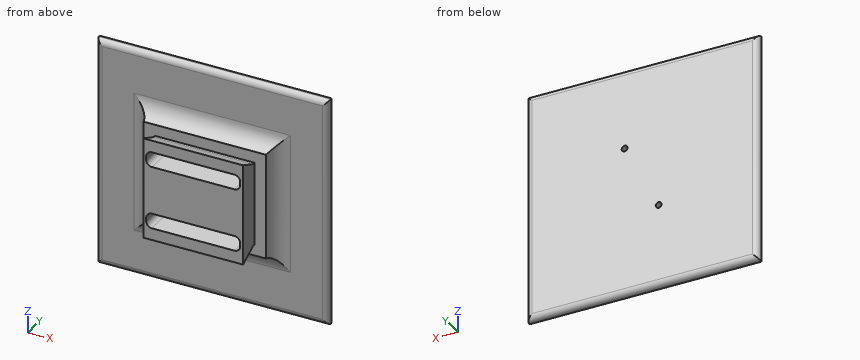
```python
from build123d import *

# Parameters (mm, degrees)
SKETCH1_W                  = 53.594
SKETCH1_H                  = 46.99
BOSS_EXTRUDE1_DEPTH        = 12.7
CUT_EXTRUDE1_DEPTH         = 62.251008522
SKETCH3_W                  = 4.953
SKETCH3_H                  = 9.653808373
CUT_EXTRUDE2_DEPTH         = 56.564640816
SKETCH4_W                  = 53.594
SKETCH4_H                  = 46.99
BOSS_EXTRUDE2_DEPTH        = 3.175
SKETCH5_W                  = 101.6
SKETCH5_H                  = 101.6
BOSS_EXTRUDE3_DEPTH        = 4.7625
FILLET1_R                  = 7.62
SKETCH6_W                  = 41.148
SKETCH6_H                  = 34.415052436
CUT_EXTRUDE3_DEPTH         = 15.875
F_2_6_2_6_DIAMETER_HOLE1_D = 2.6
FILLET2_R                  = 2.54
FILLET3_R                  = 2.54
FILLET4_R                  = 2.54
BOSS_EXTRUDE4_REACH        = 76.747
SKETCH9_W                  = 41.148
SKETCH9_H                  = 21.115558174
FILLET5_R                  = 2.54


with BuildPart() as part:
    # Sketch1 → Boss-Extrude1 (new body)
    with BuildSketch(Plane(origin=(0, 0, 0), x_dir=(1, 0, 0), z_dir=(0, 1, 0))):
        Rectangle(SKETCH1_W, SKETCH1_H)
    extrude(amount=BOSS_EXTRUDE1_DEPTH)

    # Sketch2 → Cut-Extrude1 (cut, through all)
    with BuildSketch(Plane(origin=(-26.797, 0, -3.302), x_dir=(0, 0, -1), z_dir=(1, 0, 0))):
        Polygon((-25.781, 0), (-21.779526218, 8.503564639), (-21.779526218, 9.653808373), (-26.797, 9.653808373), (-26.797, 0), align=None)
        Polygon((19.177, 0), (20.193, 0), (20.193, 9.653808373), (15.175526218, 9.653808373), (15.175526218, 8.503564639), align=None)
    extrude(amount=CUT_EXTRUDE1_DEPTH, mode=Mode.SUBTRACT)

    # Sketch3 → Cut-Extrude2 (cut, through all)
    with BuildSketch(Plane.XY.offset(23.495)):
        with Locations((-24.3205, 4.826904187)):
            Rectangle(SKETCH3_W, SKETCH3_H)
        with Locations((24.3205, 4.826904187)):
            Rectangle(SKETCH3_W, SKETCH3_H)
    extrude(amount=-CUT_EXTRUDE2_DEPTH, mode=Mode.SUBTRACT)

    # Sketch4 → Boss-Extrude2 (add)
    with BuildSketch(Plane(origin=(0, 12.7, 0), x_dir=(1, 0, 0), z_dir=(0, 1, 0))):
        Rectangle(SKETCH4_W, SKETCH4_H)
    extrude(amount=BOSS_EXTRUDE2_DEPTH)

    # Sketch5 → Boss-Extrude3 (add)
    with BuildSketch(Plane(origin=(0, 15.875, 0), x_dir=(1, 0, 0), z_dir=(0, 1, 0))):
        Rectangle(SKETCH5_W, SKETCH5_H)
    extrude(amount=BOSS_EXTRUDE3_DEPTH)

    # Fillet1
    # the kernel refuses this fillet: 7.62 mm, written as the material it adds along each edge
    with BuildSketch(Plane(origin=(-26.797, 15.875, -23.495), x_dir=(-1, 0, 0), z_dir=(0, 0, 1)), Plane(origin=(26.797, 15.875, 23.495), x_dir=(1, 0, 0), z_dir=(0, 0, -1))) as fillet1_piece_1:
        with BuildLine():
            CenterArc((7.490509671, 7.62), FILLET1_R, 190.577809731, 79.422190269)
            Line((0, 6.221191627), (-0.149810193, 6.19321546))
            ThreePointArc((-0.149810193, 6.19321546), (-0.1524, 3.110595814), (-0.1524, 0))
            Line((-0.1524, 0), (0, -0.1524))
            Line((0, -0.1524), (7.490509671, -0.1524))
            Line((7.490509671, -0.1524), (7.490509671, 0))
        make_face()
    extrude(amount=46.99)
    with BuildSketch(Plane(origin=(26.797, 15.875, -23.495), x_dir=(0, 0, -1), z_dir=(-1, 0, 0)), Plane(origin=(-26.797, 15.875, 23.495), x_dir=(0, 0, 1), z_dir=(1, 0, 0))) as fillet1_piece_2:
        with BuildLine():
            CenterArc((7.490509671, 7.62), FILLET1_R, 190.577809731, 79.422190269)
            Line((0, 6.221191627), (-0.149810193, 6.19321546))
            ThreePointArc((-0.149810193, 6.19321546), (-0.1524, 3.110595814), (-0.1524, 0))
            Line((-0.1524, 0), (0, -0.1524))
            Line((0, -0.1524), (7.490509671, -0.1524))
            Line((7.490509671, -0.1524), (7.490509671, 0))
        make_face()
    extrude(amount=53.594)
    with BuildSketch(Plane(origin=(26.797, 15.875, -23.495), x_dir=(0, 0, -1), z_dir=(-1, 0, 0))) as fillet1_piece_3a_section:
        with BuildLine():
            CenterArc((7.490509671, 7.62), FILLET1_R, 190.577809731, 79.422190269)
            Line((0, 6.221191627), (-0.149810193, 6.19321546))
            ThreePointArc((-0.149810193, 6.19321546), (-0.1524, 3.110595814), (-0.1524, 0))
            Line((-0.1524, 0), (0, -0.1524))
            Line((0, -0.1524), (7.490509671, -0.1524))
            Line((7.490509671, -0.1524), (7.490509671, 0))
        make_face()
    fillet1_piece_3a = extrude(amount=72.320274178, mode=Mode.PRIVATE)
    fillet1_piece_3a = split(fillet1_piece_3a, bisect_by=Plane(origin=(-26.797, 15.875, -23.495), z_dir=(-1, 0, 0)), keep=Keep.TOP, mode=Mode.PRIVATE)
    with BuildSketch(Plane(origin=(-26.797, 15.875, -42.221274178), x_dir=(-1, 0, 0), z_dir=(0, 0, 1))) as fillet1_piece_3b_section:
        with BuildLine():
            CenterArc((7.490509671, 7.62), FILLET1_R, 190.577809731, 79.422190269)
            Line((0, 6.221191627), (-0.149810193, 6.19321546))
            ThreePointArc((-0.149810193, 6.19321546), (-0.1524, 3.110595814), (-0.1524, 0))
            Line((-0.1524, 0), (0, -0.1524))
            Line((0, -0.1524), (7.490509671, -0.1524))
            Line((7.490509671, -0.1524), (7.490509671, 0))
        make_face()
    fillet1_piece_3b = extrude(amount=65.716274178, mode=Mode.PRIVATE)
    fillet1_piece_3b = split(fillet1_piece_3b, bisect_by=Plane(origin=(-26.797, 15.875, -23.495), z_dir=(0, 0, -1)), keep=Keep.TOP, mode=Mode.PRIVATE)
    fillet1_piece_3 = fillet1_piece_3a & fillet1_piece_3b
    add(fillet1_piece_3)
    with BuildSketch(Plane(origin=(-45.523274178, 15.875, 23.495), x_dir=(0, 0, 1), z_dir=(1, 0, 0))) as fillet1_piece_4a_section:
        with BuildLine():
            CenterArc((7.490509671, 7.62), FILLET1_R, 190.577809731, 79.422190269)
            Line((0, 6.221191627), (-0.149810193, 6.19321546))
            ThreePointArc((-0.149810193, 6.19321546), (-0.1524, 3.110595814), (-0.1524, 0))
            Line((-0.1524, 0), (0, -0.1524))
            Line((0, -0.1524), (7.490509671, -0.1524))
            Line((7.490509671, -0.1524), (7.490509671, 0))
        make_face()
    fillet1_piece_4a = extrude(amount=72.320274178, mode=Mode.PRIVATE)
    fillet1_piece_4a = split(fillet1_piece_4a, bisect_by=Plane(origin=(-26.797, 15.875, 23.495), z_dir=(-1, 0, 0)), keep=Keep.TOP, mode=Mode.PRIVATE)
    with BuildSketch(Plane(origin=(-26.797, 15.875, -23.495), x_dir=(-1, 0, 0), z_dir=(0, 0, 1))) as fillet1_piece_4b_section:
        with BuildLine():
            CenterArc((7.490509671, 7.62), FILLET1_R, 190.577809731, 79.422190269)
            Line((0, 6.221191627), (-0.149810193, 6.19321546))
            ThreePointArc((-0.149810193, 6.19321546), (-0.1524, 3.110595814), (-0.1524, 0))
            Line((-0.1524, 0), (0, -0.1524))
            Line((0, -0.1524), (7.490509671, -0.1524))
            Line((7.490509671, -0.1524), (7.490509671, 0))
        make_face()
    fillet1_piece_4b = extrude(amount=65.716274178, mode=Mode.PRIVATE)
    fillet1_piece_4b = split(fillet1_piece_4b, bisect_by=Plane(origin=(-26.797, 15.875, 23.495), z_dir=(0, 0, 1)), keep=Keep.TOP, mode=Mode.PRIVATE)
    fillet1_piece_4 = fillet1_piece_4a & fillet1_piece_4b
    add(fillet1_piece_4)
    with BuildSketch(Plane(origin=(26.797, 15.875, 23.495), x_dir=(1, 0, 0), z_dir=(0, 0, -1))) as fillet1_piece_5a_section:
        with BuildLine():
            CenterArc((7.490509671, 7.62), FILLET1_R, 190.577809731, 79.422190269)
            Line((0, 6.221191627), (-0.149810193, 6.19321546))
            ThreePointArc((-0.149810193, 6.19321546), (-0.1524, 3.110595814), (-0.1524, 0))
            Line((-0.1524, 0), (0, -0.1524))
            Line((0, -0.1524), (7.490509671, -0.1524))
            Line((7.490509671, -0.1524), (7.490509671, 0))
        make_face()
    fillet1_piece_5a = extrude(amount=65.716274178, mode=Mode.PRIVATE)
    fillet1_piece_5a = split(fillet1_piece_5a, bisect_by=Plane(origin=(26.797, 15.875, -23.495), z_dir=(0, 0, -1)), keep=Keep.TOP, mode=Mode.PRIVATE)
    with BuildSketch(Plane(origin=(45.523274178, 15.875, -23.495), x_dir=(0, 0, -1), z_dir=(-1, 0, 0))) as fillet1_piece_5b_section:
        with BuildLine():
            CenterArc((7.490509671, 7.62), FILLET1_R, 190.577809731, 79.422190269)
            Line((0, 6.221191627), (-0.149810193, 6.19321546))
            ThreePointArc((-0.149810193, 6.19321546), (-0.1524, 3.110595814), (-0.1524, 0))
            Line((-0.1524, 0), (0, -0.1524))
            Line((0, -0.1524), (7.490509671, -0.1524))
            Line((7.490509671, -0.1524), (7.490509671, 0))
        make_face()
    fillet1_piece_5b = extrude(amount=72.320274178, mode=Mode.PRIVATE)
    fillet1_piece_5b = split(fillet1_piece_5b, bisect_by=Plane(origin=(26.797, 15.875, -23.495), z_dir=(1, 0, 0)), keep=Keep.TOP, mode=Mode.PRIVATE)
    fillet1_piece_5 = fillet1_piece_5a & fillet1_piece_5b
    add(fillet1_piece_5)
    with BuildSketch(Plane(origin=(-26.797, 15.875, 23.495), x_dir=(0, 0, 1), z_dir=(1, 0, 0))) as fillet1_piece_6a_section:
        with BuildLine():
            CenterArc((7.490509671, 7.62), FILLET1_R, 190.577809731, 79.422190269)
            Line((0, 6.221191627), (-0.149810193, 6.19321546))
            ThreePointArc((-0.149810193, 6.19321546), (-0.1524, 3.110595814), (-0.1524, 0))
            Line((-0.1524, 0), (0, -0.1524))
            Line((0, -0.1524), (7.490509671, -0.1524))
            Line((7.490509671, -0.1524), (7.490509671, 0))
        make_face()
    fillet1_piece_6a = extrude(amount=72.320274178, mode=Mode.PRIVATE)
    fillet1_piece_6a = split(fillet1_piece_6a, bisect_by=Plane(origin=(26.797, 15.875, 23.495), z_dir=(1, 0, 0)), keep=Keep.TOP, mode=Mode.PRIVATE)
    with BuildSketch(Plane(origin=(26.797, 15.875, 42.221274178), x_dir=(1, 0, 0), z_dir=(0, 0, -1))) as fillet1_piece_6b_section:
        with BuildLine():
            CenterArc((7.490509671, 7.62), FILLET1_R, 190.577809731, 79.422190269)
            Line((0, 6.221191627), (-0.149810193, 6.19321546))
            ThreePointArc((-0.149810193, 6.19321546), (-0.1524, 3.110595814), (-0.1524, 0))
            Line((-0.1524, 0), (0, -0.1524))
            Line((0, -0.1524), (7.490509671, -0.1524))
            Line((7.490509671, -0.1524), (7.490509671, 0))
        make_face()
    fillet1_piece_6b = extrude(amount=65.716274178, mode=Mode.PRIVATE)
    fillet1_piece_6b = split(fillet1_piece_6b, bisect_by=Plane(origin=(26.797, 15.875, 23.495), z_dir=(0, 0, 1)), keep=Keep.TOP, mode=Mode.PRIVATE)
    fillet1_piece_6 = fillet1_piece_6a & fillet1_piece_6b
    add(fillet1_piece_6)

    # Sketch6 → Cut-Extrude3 (cut)
    with BuildSketch(Plane.XZ):
        Rectangle(SKETCH6_W, SKETCH6_H)
    extrude(amount=-CUT_EXTRUDE3_DEPTH, mode=Mode.SUBTRACT)

    # Ø2.6 (2.6) Diameter Hole1 (through all)
    with Locations(Plane(origin=(0, 20.6375, 0), x_dir=(1, 0, 0), z_dir=(0, 1, 0))):
        with Locations((-7.25, 14.6), (7.65, -15.1)):
            Hole(F_2_6_2_6_DIAMETER_HOLE1_D / 2)

    # Fillet2
    fillet2_edges = [part.edges().sort_by_distance(p)[0] for p in [
        (50.8, 20.6375, 0),
        (0, 20.6375, -50.8),
        (-50.8, 20.6375, 0),
        (0, 20.6375, 50.8),
    ]]
    fillet(fillet2_edges, radius=FILLET2_R)

    # Fillet3
    # the kernel refuses this fillet: 2.54 mm, written as the material it takes off along each edge
    with BuildSketch(Plane(origin=(57.100195309, 15.875, -50.8), x_dir=(0, 0, 1), z_dir=(-1, 0, 0)), Plane(origin=(50.8, 15.875, 57.100195309), x_dir=(-1, 0, 0), z_dir=(0, 0, -1))) as fillet3_piece_1:
        with BuildLine():
            CenterArc((2.520078124, 2.54), FILLET3_R, 187.180755781, 82.819244219)
            Line((0, 2.2225), (-0.050401562, 2.21615))
            ThreePointArc((-0.050401562, 2.21615), (-0.0508, 1.11125), (-0.0508, 0))
            Line((-0.0508, 0), (0, -0.0508))
            Line((0, -0.0508), (2.520078124, -0.0508))
            Line((2.520078124, -0.0508), (2.520078124, 0))
        make_face()
    extrude(amount=114.200390619, mode=Mode.SUBTRACT)
    with BuildSketch(Plane(origin=(-50.8, 15.875, -57.100195309), x_dir=(0, 1, 0), z_dir=(0, 0, 1)), Plane(origin=(-57.100195309, 15.875, 50.8), x_dir=(0, 1, 0), z_dir=(1, 0, 0))) as fillet3_piece_2:
        with BuildLine():
            CenterArc((2.54, -2.520078124), FILLET3_R, 97.180755781, 82.819244219)
            Line((0, -2.520078124), (-0.0508, -2.520078124))
            Line((-0.0508, -2.520078124), (-0.0508, 0))
            Line((-0.0508, 0), (0, 0.0508))
            ThreePointArc((0, 0.0508), (1.11125, 0.0508), (2.21615, 0.050401562))
            Line((2.21615, 0.050401562), (2.2225, 0))
        make_face()
    extrude(amount=114.200390619, mode=Mode.SUBTRACT)

    # Fillet4
    fillet4_edges = [part.edges().sort_by_distance(p)[0] for p in [
        (20.574, 7.9375, 17.207526218),
        (20.574, 7.9375, -17.207526218),
        (-20.574, 7.9375, -17.207526218),
        (-20.574, 7.9375, 17.207526218),
    ]]
    fillet(fillet4_edges, radius=FILLET4_R)

    # Sketch9 → Boss-Extrude4 (add, up to next)
    with BuildSketch(Plane.XZ, mode=Mode.PRIVATE) as boss_extrude4_sk1:
        Rectangle(SKETCH9_W, SKETCH9_H)
    boss_extrude4_tool1 = extrude(boss_extrude4_sk1.sketch, amount=-BOSS_EXTRUDE4_REACH, mode=Mode.PRIVATE) - part.part
    add(boss_extrude4_tool1.solids().sort_by_distance((0, 0, 0))[0])

    # Fillet5
    fillet5_edges = [part.edges().sort_by_distance(p)[0] for p in [
        (-20.574, 7.9375, 10.557779087),
        (20.574, 7.9375, -10.557779087),
        (-20.574, 7.9375, -10.557779087),
        (20.574, 7.9375, 10.557779087),
    ]]
    fillet(fillet5_edges, radius=FILLET5_R)


solid = part.part
```
Here's how the part is built. I have some questions about the finished solid (model axes, mm). Coordinates: 2 decimals unless noted, no trailing zeros. Loops run counter-clockwise (first coordinate to the right, second up) from the corner with the lowest first, then second, coordinate; pieces in that order, holes last. Notation, with made-up numbers: (74, -8.5) - (129, -8.5) arc R7 cw to (129, -1.5) - close; hole circle Ø8 at (47, 57). An arc over 180 degrees is marked (long way). Return JSON: item names as keys, results as strings. Group by question number.
Item 1: I need wall thicknesses on line 1 (X direction, y = 17.95, z = -14.6); line 2 (Z direction, x = -18, y = 5.5); line 3 (Y direction, x = 8, z = 12) (1 decimal). Which ranges of each line are inside material? Lowest first, please. Write a range as from..to.
Item 2: If we section it at B-B on z = -5: Write out the boundary of the cut face in (x, y) (1 decimal), and give its area (3 significant figures).
Item 3: If we section it at C-C on y = 5.75: Write out the boundary of the cut face in (x, z), and give its area (3 significant figures).
Item 4: If we section it at A-A on x = -7.25: Write out the boundary of the cut face in (y, z) (1 decimal), and give its area (3 significant figures).
Item 5: If we section it at D-D on x = 15.5: Write out the boundary of the cut face in (y, z) (1 decimal), and give its area (3 significant figures).
Item 6: Will these pins go through, and if not, where does the flat tip stop? P1, Ø2.5, axis at x = 7.65, z = 15.1, coming from the -Y side; P2, Ø12, axis at y = 11, z = -24.5, coming from the +X side; P3, Ø5.5, axis at x = -9.5, z = 13.5, coming from the -Y side (3 decimals); P4, Ø1.7, axis at y = 6, z = 13.5, coming from the -X side.
Calculated:
{
 "1": {"line 1": "x = -50.78..-8.55, -5.95..50.78", "line 2": "z = -19.89..-17.21, -10.56..10.56, 17.21..19.89", "line 3": "y = 15.9..20.6"},
 "2": {"outline": "(-50.8, 18.1) arc R2.5 ccw to (-48.3, 15.9) - (-34.3, 15.9) arc R7.6 cw to (-26.8, 9.7) - (-21.8, 9.7) - (-21.8, 0) - (21.8, 0) - (21.8, 9.7) - (26.8, 9.7) arc R7.6 cw to (34.3, 15.9) - (48.3, 15.9) arc R2.5 ccw to (50.8, 18.1) arc R2.5 ccw to (48.3, 20.6) - (-48.3, 20.6) arc R2.5 ccw to start", "area": "1,260 mm^2"},
 "3": {"outline": "(-21.84, -19.77) - (21.84, -19.77) - (21.84, 19.77) - (-21.84, 19.77) - close; hole (-20.57, -14.67) arc R2.54 ccw to (-18.03, -17.21) - (18.03, -17.21) arc R2.54 ccw to (20.57, -14.67) - (20.57, -13.1) arc R2.54 ccw to (18.03, -10.56) - (-18.03, -10.56) arc R2.54 ccw to (-20.57, -13.1) - close; hole (-20.57, 13.1) arc R2.54 ccw to (-18.03, 10.56) - (18.03, 10.56) arc R2.54 ccw to (20.57, 13.1) - (20.57, 14.67) arc R2.54 ccw to (18.03, 17.21) - (-18.03, 17.21) arc R2.54 ccw to (-20.57, 14.67) - close", "area": "1,190 mm^2"},
 "4": {"outline": "(0, -22.5) - (8.5, -18.5) - (9.7, -18.5) - (9.7, -23.5) arc R7.6 cw to (15.9, -31) - (15.9, -48.3) arc R2.5 ccw to (18.1, -50.8) arc R2.5 ccw to (20.6, -48.3) - (20.6, -15.9) - (15.9, -15.9) - (15.9, -17.2) - (0, -17.2) - close; (0, -10.6) - (15.9, -10.6) - (15.9, -13.3) - (20.6, -13.3) - (20.6, 48.3) arc R2.5 ccw to (18.1, 50.8) arc R2.5 ccw to (15.9, 48.3) - (15.9, 31) arc R7.6 cw to (9.7, 23.5) - (9.7, 18.5) - (8.5, 18.5) - (0, 22.5) - (0, 17.2) - (15.9, 17.2) - (15.9, 10.6) - (0, 10.6) - close", "area": "961 mm^2"},
 "5": {"outline": "(0, -22.5) - (8.5, -18.5) - (9.7, -18.5) - (9.7, -23.5) arc R7.6 cw to (15.9, -31) - (15.9, -48.3) arc R2.5 ccw to (18.1, -50.8) arc R2.5 ccw to (20.6, -48.3) - (20.6, 48.3) arc R2.5 ccw to (18.1, 50.8) arc R2.5 ccw to (15.9, 48.3) - (15.9, 31) arc R7.6 cw to (9.7, 23.5) - (9.7, 18.5) - (8.5, 18.5) - (0, 22.5) - (0, 17.2) - (15.9, 17.2) - (15.9, 10.6) - (0, 10.6) - (0, -10.6) - (15.9, -10.6) - (15.9, -17.2) - (0, -17.2) - close", "area": "974 mm^2"},
 "6": {"P1": "passes through", "P2": "stops at x = 50.39", "P3": "stops at y = 15.875", "P4": "stops at x = -21.84"}
}
